Model file for the job. Use its own axes, mm. A direction names the side the tool comes from. Give positions to 0.01 mm unless a question says otherwise; leave off trailing zeros. Write each loop counter-clockwise with the first axis right and the second up, starting at its lowest first coordinate (ties: lowest second). Pieces come first, ordered by that corner, then holes.
```python
from build123d import *

# Parameters (mm, degrees)
SKETCH1_W           = 48
SKETCH1_H           = 35
BOSS_EXTRUDE1_DEPTH = 1
SKETCH2_W           = 48
SKETCH2_H           = 1
BOSS_EXTRUDE2_DEPTH = 17
FILLET1_R           = 1
SKETCH3_R           = 1.35
SKETCH3_R_2         = 15
CUT_EXTRUDE1_DEPTH  = 35.731109974
SKETCH4_W           = 48
SKETCH4_H           = 1
BOSS_EXTRUDE3_DEPTH = 15
SKETCH5_R           = 1
SKETCH5_W           = 20
SKETCH5_H           = 10
CUT_EXTRUDE2_DEPTH  = 45.229515032
FILLET2_R           = 1
SKETCH6_R           = 1.5
CUT_EXTRUDE3_DEPTH  = 58.148928249
FILLET3_R           = 5


with BuildPart() as part:
    # Sketch1 → Boss-Extrude1 (new body)
    with BuildSketch(Plane.XY):
        Rectangle(SKETCH1_W, SKETCH1_H)
    extrude(amount=BOSS_EXTRUDE1_DEPTH)

    # Sketch2 → Boss-Extrude2 (add)
    with BuildSketch(Plane(origin=(0, 0, 0), x_dir=(-1, 0, 0), z_dir=(0, 0, -1))):
        with Locations((0, -17)):
            Rectangle(SKETCH2_W, SKETCH2_H)
    extrude(amount=BOSS_EXTRUDE2_DEPTH)

    # Fillet1
    fillet1_edges = [part.edges().sort_by_distance(p)[0] for p in [
        (0, -16.5, 0),
    ]]
    fillet(fillet1_edges, radius=FILLET1_R)

    # Sketch3 → Cut-Extrude1 (cut, through all)
    with BuildSketch(Plane.XY.offset(1)):
        with Locations((-21, 10)):
            Circle(SKETCH3_R)
        Circle(SKETCH3_R_2)
        with Locations((-21, -8)):
            Circle(SKETCH3_R)
        with Locations((21, -8)):
            Circle(SKETCH3_R)
        with Locations((21, 10)):
            Circle(SKETCH3_R)
    extrude(amount=-CUT_EXTRUDE1_DEPTH, mode=Mode.SUBTRACT)

    # Sketch4 → Boss-Extrude3 (add)
    with BuildSketch(Plane(origin=(0, 17.5, 0), x_dir=(1, 0, 0), z_dir=(0, 1, 0))):
        with Locations((0, -0.5)):
            Rectangle(SKETCH4_W, SKETCH4_H)
    extrude(amount=BOSS_EXTRUDE3_DEPTH)

    # Sketch5 → Cut-Extrude2 (cut, through all)
    with BuildSketch(Plane.XY.offset(1)):
        with Locations((-19, 26)):
            Circle(SKETCH5_R)
        with Locations((19, 26)):
            Circle(SKETCH5_R)
        with Locations((0, 26)):
            Rectangle(SKETCH5_W, SKETCH5_H)
    extrude(amount=-CUT_EXTRUDE2_DEPTH, mode=Mode.SUBTRACT)

    # Fillet2
    fillet2_edges = [part.edges().sort_by_distance(p)[0] for p in [
        (10, 31, 0.5),
        (10, 21, 0.5),
        (-10, 21, 0.5),
        (-10, 31, 0.5),
    ]]
    fillet(fillet2_edges, radius=FILLET2_R)

    # Sketch6 → Cut-Extrude3 (cut, through all)
    with BuildSketch(Plane(origin=(0, -16.5, 0), x_dir=(1, 0, 0), z_dir=(0, 1, 0))):
        with Locations(Location((21, 5, 0), (0, 0, 270))):
            Circle(SKETCH6_R)
        with Locations(Location((21, 14, 0), (0, 0, 270))):
            Circle(SKETCH6_R)
        with Locations(Location((-21, 5, 0), (0, 0, 90))):
            Circle(SKETCH6_R)
        with Locations(Location((-21, 14, 0), (0, 0, 90))):
            Circle(SKETCH6_R)
    extrude(amount=-CUT_EXTRUDE3_DEPTH, mode=Mode.SUBTRACT)

    # Fillet3
    fillet3_edges = [part.edges().sort_by_distance(p)[0] for p in [
        (24, 32.5, 0.5),
        (-24, 32.5, 0.5),
    ]]
    fillet(fillet3_edges, radius=FILLET3_R)


solid = part.part
```
1. Probe probe 1 along Z at (x, y) = (-21, -17.15); probe 2 along Y at (x, z) = (0, 0.2); probe 3 along X at (y, z) = (-17.15, -5). List the from-to ranges inside material, lowest first.
Calculated:
probe 1: z = -17 to -15.5, -12.5 to -6.5, -3.5 to 1
probe 2: y = -17.5 to -15, 15 to 21, 31 to 32.5
probe 3: x = -24 to -22.5, -19.5 to 19.5, 22.5 to 24
2. Pull direction Y, two halves, no side cores. Call faces 3 (the cylindrical face through (-20.274, -6.862, 0.507)), 4 (the cylindrical face through (-22.57, 31, 0.49)), 5 (the cylindrical face through (-22.265, -16.993, -5.806)): +Y half, -Y half, draft (parallel to the pull), parting line (faces both ways), or undercut.
Calculated:
face 3: undercut
face 4: +Y half
face 5: draft
3. Slice it at A-A, the plane y = 26. Write the cut outline in (x, z).
Calculated:
outline: (-24, 0) - (-20, 0) - (-20, 1) - (-24, 1) - close; (-18, 0) - (-10, 0) - (-10, 1) - (-18, 1) - close; (10, 0) - (18, 0) - (18, 1) - (10, 1) - close; (20, 0) - (24, 0) - (24, 1) - (20, 1) - close
4. Slice it at C-C, the plane x = 0. Write the cut outline in (y, z).
Calculated:
outline: (-17.5, -17) - (-16.5, -17) - (-16.5, -1) arc R1 cw to (-15.5, 0) - (-15, 0) - (-15, 1) - (-17.5, 1) - close; (15, 0) - (21, 0) - (21, 1) - (15, 1) - close; (31, 0) - (32.5, 0) - (32.5, 1) - (31, 1) - close
5. Slice it at B-B, the plane z = -14. Write the cut outline in (x, y), and give its area (3 significant figures).
Calculated:
outline: (-24, -17.5) - (-22.5, -17.5) - (-22.5, -16.5) - (-24, -16.5) - close; (-19.5, -17.5) - (19.5, -17.5) - (19.5, -16.5) - (-19.5, -16.5) - close; (22.5, -17.5) - (24, -17.5) - (24, -16.5) - (22.5, -16.5) - close
area: 42.0 mm2
6. Pin check, flat tips, straight feed: P1, Ø14.5, axis at x = 10.5, y = 18.5, coming from the -Z side; P2, Ø8, axis at x = -17, z = -10, coming from the +Y side. Stop position of each tip, or through.
Calculated:
P1: stops at z = 0
P2: stops at y = -16.5
7. Which spindle directions (+Z, -Z, +X, -X, +Y, -Y) get a long thin tool onto all of the face, cutting with end or side? Do faces 1 (the cylindrical face through (-19.8, 25.4, 0.5)), 2 (the flat face through (0, 19, 0)). Say none if no direction does.
Calculated:
face 1: +Z, -Z
face 2: -Z, +X, -X, +Y
8. Slice it at D-D, the plane y = 0. Write the cut outline in (x, z), and give its area (3 significant figures).
Calculated:
outline: (-24, 0) - (-15, 0) - (-15, 1) - (-24, 1) - close; (15, 0) - (24, 0) - (24, 1) - (15, 1) - close
area: 18.0 mm2
